Here's how the part is built. I have some questions about the finished solid (model axes, mm). A direction names the side the tool comes from. Round coordinates to 2 decimals unless told otherwise and drop trailing zeros. Write each loop counter-clockwise with the first axis right and the second up, starting at its lowest first coordinate (ties: lowest second). Pieces come first, ordered by that corner, then holes. Notation, with made-up numbers: (58.25, 74) -> (90.25, 74) arc R13 ccw to (90.25, 99) -> close; hole circle Ø9 at (-36, 47.5). An arc over 180 degrees is marked (long way). Put each result on its own line as item: value. Start each with the question number.
1. For pin 1 (6 mm diameter, centred on y = 8.5, z = 6.5, fed in from +X) (3 decimals); pin 2 (17 mm diameter, centred on x = 0, y = 0, fed in from +Z); pin 3 (6 mm diameter, centred on x = -7.5, z = 5, fed in from -Y), each with a flat end and sliding along its axis, tell me the tip position at first contact or that it passes through.
2. I need wall thicknesses on probe 1 along Y at (x, z) = (0, 0.55); probe 2 along Y at (x, z) = (0, 7); probe 3 along Z at (x, y) = (2, 12). Which ranges of each line are inside material? Lowest first, please. Write a range as from..to.
3. Suppose I cut it at D-D (x = 9). Please give me the cut outline in (y, z).
4. Which directions (+Z, -Z, +X, -X, +Y, -Y) give clear straight access to the entire face, cutting with the end or side of a thin tool? Please do faces 4 (the face through (-6, 0, 1)), 5 (the face through (3, -6, 2)).
5. Suppose I cut it at A-A (x = 0). Please give me the cut outline in (y, z), then the cut area to 3 significant figures.
6. Suppose I cut it at C-C (z = 4). Please give me the cut outline in (x, y), then the cut area to 3 significant figures.
7. We'd pull the mould along X, two halves only. Please class faces 1 (the face through (-0.07, -14.15, 10)), 2 (the face through (-3.47, -15.62, 4.93)), 3 (the face through (12.932, -5.362, 5.944)): +X half, -X half, draft (parallel to the pull), parting line (faces both ways), or undercut.
```python
from build123d import *

# Parameters (mm, degrees)
CYLINDER002_R     = 6
CYLINDER002_DEPTH = 10
CYLINDER_R        = 14
CYLINDER_DEPTH    = 13
CYLINDER001_R     = 16
CYLINDER001_DEPTH = 10


with BuildPart() as cylinder002:
    # Cylinder002 → Cylinder002 (new body)
    with BuildSketch(Plane.XY):
        Circle(CYLINDER002_R)
    extrude(amount=CYLINDER002_DEPTH)


with BuildPart() as cylinder:
    # Cylinder → Cylinder (new body)
    with BuildSketch(Plane.XY.offset(2)):
        Circle(CYLINDER_R)
    extrude(amount=CYLINDER_DEPTH)


with BuildPart() as cut001:
    # Cylinder001 → Cylinder001 (new body)
    with BuildSketch(Plane.XY):
        Circle(CYLINDER001_R)
    extrude(amount=CYLINDER001_DEPTH)

    # Cut: cut Cylinder
    add(cylinder.part, mode=Mode.SUBTRACT)

    # Cut001: cut Cylinder002
    add(cylinder002.part, mode=Mode.SUBTRACT)


solid = cut001.part
```
Verdict:
1. pin 1: stops at x = 15.025
1. pin 2: stops at z = 2
1. pin 3: stops at y = -15.35
2. probe 1: y = -16..-6, 6..16
2. probe 2: y = -16..-14, 14..16
2. probe 3: z = 0..2
3. outline: (-13.23, 0) -> (13.23, 0) -> (13.23, 10) -> (10.72, 10) -> (10.72, 2) -> (-10.72, 2) -> (-10.72, 10) -> (-13.23, 10) -> close
4. face 4: +Z, -Z
4. face 5: +Z
5. outline: (-16, 0) -> (-6, 0) -> (-6, 2) -> (-14, 2) -> (-14, 10) -> (-16, 10) -> close; (6, 0) -> (16, 0) -> (16, 10) -> (14, 10) -> (14, 2) -> (6, 2) -> close
5. area: 72.0 mm^2
6. outline: circle Ø32 at (0, 0); hole circle Ø28 at (0, 0)
6. area: 188 mm^2
7. face 1: draft
7. face 2: parting line
7. face 3: undercut
